Design review of the part built by this model. Coordinates are the model's own, in mm. A direction names the side the tool comes from. Round coordinates to 2 decimals unless told otherwise and drop trailing zeros. Loops run counter-clockwise (first coordinate to the right, second up) from the corner with the lowest first, then second, coordinate; pieces in that order, holes last. Notation, with made-up numbers: M -26,54.5 L 20,54.5 A15 cw 20,62.5 Z; hole C 26.25,-23.5 d3. An arc over 180 degrees is marked long. Use a Markdown table: item, result.
from build123d import *

# Parameters (mm, degrees)
SKETCH1_W                = 600
SKETCH1_H                = 50
BASE_FLANGE1_DEPTH       = 1.5
SKETCHED_START           = -300
SKETCHED_BEND2_DEPTH     = 600
SKETCHED_BEND2_2_DEPTH   = 600
F_4_0_4_DIAMETER_HOLE1_D = 4
F_5_0_5_DIAMETER_HOLE1_D = 5
CUT_EXTRUDE1_REACH       = 304.135
SKETCH11_W               = 102
SKETCH11_H               = 16


# Read off the part's stored shape, not the designer's step: Sketched Bend2
# Sheet-metal steps are written as plain solids
with BuildPart() as part:
    # Sketch1 → Base-Flange1 (new body)
    with BuildSketch(Plane.YZ):
        Rectangle(SKETCH1_W, SKETCH1_H)
    extrude(amount=-BASE_FLANGE1_DEPTH)

    # Sketched Bend2 outline → Sketched Bend2 (cut)
    with BuildSketch(Plane(origin=(0, 0, 0), x_dir=(1, 0, 0), z_dir=(0, 1, 0)).offset(SKETCHED_START)):
        with BuildLine():
            Line((0, -25), (0, 1.686367809))
            ThreePointArc((0, 1.686367809), (-1.098076211, 2.78444402), (-1.5, 4.28444402))
            Line((-1.5, 4.28444402), (-1.5, -25))
            Line((-1.5, -25), (0, -25))
        make_face()
    extrude(amount=SKETCHED_BEND2_DEPTH, mode=Mode.SUBTRACT)

    # Sketched Bend2 2 outline → Sketched Bend2 2 (add)
    with BuildSketch(Plane(origin=(0, 0, 0), x_dir=(1, 0, 0), z_dir=(0, 1, 0)).offset(SKETCHED_START)):
        with BuildLine():
            Line((2.52606043, 1.465366158), (25.985255658, 10.003814941))
            Line((25.985255658, 10.003814941), (25.472225443, 11.413353872))
            Line((25.472225443, 11.413353872), (2.013030215, 2.874905089))
            ThreePointArc((2.013030215, 2.874905089), (0.639635346, 3.055715954), (0, 4.28444402))
            Line((0, 4.28444402), (0, 1.686367809))
            ThreePointArc((0, 1.686367809), (1.238532772, 1.295859926), (2.52606043, 1.465366158))
        make_face()
    extrude(amount=SKETCHED_BEND2_2_DEPTH)

    # Ø4.0 (4) Diameter Hole1 (through all)
    with Locations(Plane(origin=(-0.175466668, 0, -0.482090707), x_dir=(0, -1, 0), z_dir=(0.3420201433256727, 0, 0.9396926207859071))):
        with Locations((287.3, 15.139659211), (12.7, 15.139659211)):
            f_4_0_4_diameter_hole1 = Hole(F_4_0_4_DIAMETER_HOLE1_D / 2)

    # Mirror1: Ø4.0 (4) Diameter Hole1 across plane
    add(f_4_0_4_diameter_hole1.mirror(Plane.ZX), mode=Mode.SUBTRACT)

    # Ø5.0 (5) Diameter Hole1 (through all)
    with Locations(Plane(origin=(-1.5, 0, 0), x_dir=(0, -1, 0), z_dir=(-1, 0, 0))):
        with Locations((-287.3, -16.98444402), (-87.3, -16.98444402), (87.3, -16.98444402), (287.3, -16.98444402)):
            Hole(F_5_0_5_DIAMETER_HOLE1_D / 2)

    # Sketch11 → Cut-Extrude1 (cut, up to next)
    with BuildSketch(Plane(origin=(-0.175466668, 0, -0.482090707), x_dir=(0, -1, 0), z_dir=(0.3420201433256727, 0, 0.9396926207859071)), mode=Mode.PRIVATE) as cut_extrude1_sk1:
        with Locations((218, 19.839659211)):
            Rectangle(SKETCH11_W, SKETCH11_H)
    cut_extrude1_tool1 = extrude(cut_extrude1_sk1.sketch, amount=-CUT_EXTRUDE1_REACH, mode=Mode.PRIVATE) & part.part
    add(cut_extrude1_tool1.solids().sort_by_distance((18.467715, -218, -7.267654))[0], mode=Mode.SUBTRACT)


solid = part.part
1. Machinability: for faces 1 (the face through (13.9, -4.2, -7.2)), 2 (the face through (14.091, -4.2, -5.675)), which of the approach directions +Z, -Z, +X, -X, +Y, -Y give a long, thin tool a straight path to every point of the face, cutting with its end or side? Answer none if there is none.
Check values:
| item | result |
|---|---|
| face 1 | -Z, +Y, -Y |
| face 2 | +Z, +X, +Y, -Y |
2. Wall thickness on line 1 along X through (y, z) = (-245.5, -13.25); line 2 along Z through (x, y) = (-0.4, 87.3); line 3 along Z through (x, y) = (-0.9, 287.3): over which ranges is each line inside the solid? List them lowest first. Write a range as from..to.
Check values:
| item | result |
|---|---|
| line 1 | x = -1.5..0 |
| line 2 | z = -25..-19.48, -14.48..-1.96 |
| line 3 | z = -25..-19.48, -14.48..-2.48 |
3. Take a section at A-A on y = 131. Give the boundary of the cut face in (x, z).
Check values:
| item | result |
|---|---|
| outline | M -1.5,-25 L 0,-25 L 0,-4.28 A1.5 cw 2.01,-2.87 L 25.47,-11.41 L 25.99,-10 L 2.53,-1.47 A3 ccw -1.5,-4.28 Z |
4. The part is to be moulded in two halves that separate along X. For faces 3 (the face through (0, -4, -14)), 4 (the face through (7, -300, -4)), 5 (the face through (-1.5, -4, -14)), say which applies: pulls with the +X half, pulls with the -X half, needs draft (parallel to the pull), parting line crosses it, or undercut.
Check values:
| item | result |
|---|---|
| face 3 | undercut |
| face 4 | needs draft |
| face 5 | pulls with the -X half |
5. Insertion check: pin 1 (4 mm diameter, centred on x = 19, y = 187.5, fed in from -Z); pin 2 (7.5 mm diameter, centred on x = 19, z = -7, fed in from -Y); pin 3 (6 mm diameter, centred on y = 87.3, z = -16.98, fed in from +X); pin 4 (12 mm diameter, centred on y = 140.5, z = -10, fed in from +X). Each pin has a flat end and moves straight along its axis. Give the tip position at first contact, or say it passes through.
Check values:
| item | result |
|---|---|
| pin 1 | stops at z = -9.79 |
| pin 2 | stops at y = -300 |
| pin 3 | stops at x = 0 |
| pin 4 | stops at x = 25.99 |
